Source: three-view drawing plus pictorial views. Frame: mm from the lowest corner of the part. A direction names the side the tool comes from. Coordinates: 2 decimals unless noted, no trailing zeros. Loops run counter-clockwise (first coordinate to the right, second up) from the corner with the lowest first, then second, coordinate; pieces in that order, holes last.
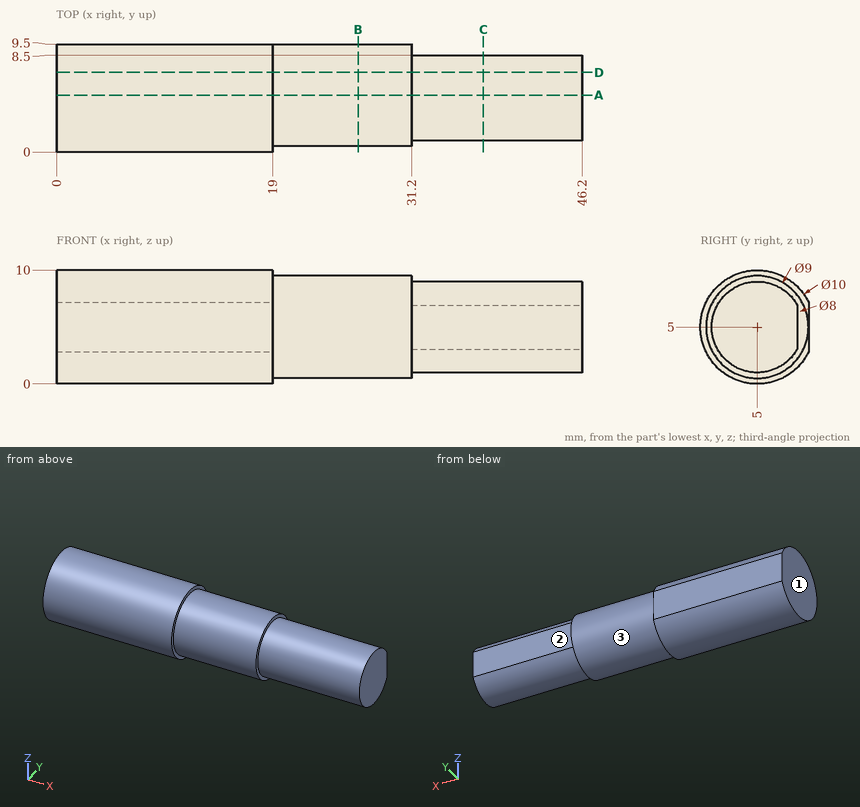
Q1. Reachability of the marked faces 1, 2 and 3 from +Z, -Z, +X, -X, +Y, -Y: full face, straight path, thin tool, end or side. Return the list, or none.
Q2. Section query A-A on y = 5. Return the cut outline in (x, z), then the cut area to 3 significant figures.
Q3. Section query C-C on x = 37.5. Return the cut outline in (y, z), then the cut area to 3 significant figures.
Q4. Section query B-B on x = 26.5. Return the cut outline in (y, z), then the cut area to 3 significant figures.
Q5. Section query D-D on y = 7. Return the cut outline in (x, z), then the cut area to 3 significant figures.
Q6. Material intervals for line 1 along X through (y, z) = (6.75, 1); line 2 along Z through (x, y) = (36, 5.25); line 3 along Y through (x, z) = (38, 1.5), sorted ascending.
Q7. First-contact query: pin 1 Ø1.5 at (y, z) = (5.5, 4) entering from -X; pin 2 Ø3 at (x, z) = (22, 5.5) entering from -Y; pin 3 Ø1 at (x, z) = (27, 3) entering from +Y; pin 4 Ø5 at (x, y) = (26.5, 1) entering from -Z. Flat tips, straight axial feed; report the tip coordinate or a pass-through.
Resolved:
1. face 1: +Z, -Z, -X, +Y, -Y
1. face 2: +Z, -Z, +X, +Y
1. face 3: +X
2. outline: (0, 0) - (19, 0) - (19, 0.5) - (31.2, 0.5) - (31.2, 1) - (46.2, 1) - (46.2, 9) - (31.2, 9) - (31.2, 9.5) - (19, 9.5) - (19, 10) - (0, 10) - close
2. area: 420 mm2
3. outline: (8.5, 3.06) - (8.5, 6.94) arc R4 ccw (long way) to start
3. area: 49.0 mm2
4. outline: circle Ø9 at (5, 5)
4. area: 63.6 mm2
5. outline: (0, 0.42) - (19, 0.42) - (19, 0.97) - (31.2, 0.97) - (31.2, 1.54) - (46.2, 1.54) - (46.2, 8.46) - (31.2, 8.46) - (31.2, 9.03) - (19, 9.03) - (19, 9.58) - (0, 9.58) - close
5. area: 376 mm2
6. line 1: x = 0 to 31.2
6. line 2: z = 1.01 to 8.99
6. line 3: y = 3.06 to 6.94
7. pin 1: stops at x = 0
7. pin 2: stops at y = 0.5
7. pin 3: stops at y = 9.24
7. pin 4: stops at z = 0.76
